Autodesk Inventor part; units mm, degrees
ref_plane "YZ Plane" through (0, 0, 0) normal (1, 0, 0) x (0, 1, 0)
ref_plane "XZ Plane" through (0, 0, 0) normal (0, 1, 0) x (-1, 0, 0)
ref_plane "XY Plane" through (0, 0, 0) normal (0, 0, 1) x (1, 0, 0)
sketch "Sketch1" plane through (0, 0, 0) normal (0, 0, 1) x (1, 0, 0)
  line L0 (0, 0) -> (0, 39.4806) construction
  line L1 (0, 0) -> (-3, 0) construction
  line L2 (-3, 0) -> (-3, 27)
  line L3 (-3, 27) -> (-5, 27)
  line L4 (-5, 27) -> (-5, 28.75)
  line L5 (0, 0) -> (0, 29)
  line L6 (-3, 0) -> (-2.65, 0)
  line L7 (-2.65, -1.5) -> (0, -1.5)
  line L8 (0, -1.5) -> (0, 0)
  line L9 (-2.65, 0) -> (-2.65, -1.5)
  line L10 (-5, 28.75) -> (0, 28.75)
  dimension "d0" = 3
  dimension "d1" = 5
  dimension "d5" = 27
  dimension "d12" = 2.65
  dimension "d13" = 1.5
  dimension "d24" = 1.75
revolve "Revolution1" add sketch "Sketch1" angle 360 about axis through (0, 0, 0) along (0, 1, 0)
sketch "Sketch3" plane through (0, -1.5, 0) normal (0, -1, 0) x (1, 0, 0)
  point P0 (0, 0)
  point P1 (0, 0)
hole "Hole1" at (0, -1.5, 0) direction (0, 1, 0) diameter 3.242 depth 11.8 tip angle 118
sketch "Sketch4" plane through (0, 27, 0) normal (0, -1, 0) x (1, 0, 0)
  arc A0 (4, 3) -> (-4, 3) centre (0, 0) ccw
  line L0 (-4, 3) -> (4, 3)
  circle A1 centre (0, 0) radius 3
  circle A2 centre (0, 0) radius 5
extrude "Extrusion2" cut sketch "Sketch4" against normal through all contours L0 A0
properties part number "shim_peg_V3"
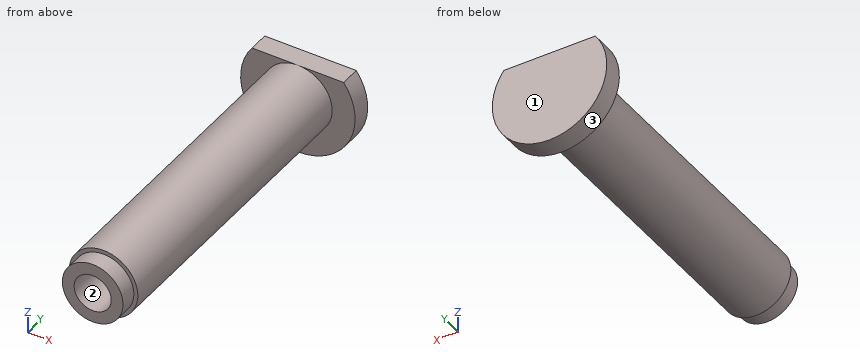
Part model, mm, in its own coordinate system. Face numbers are marked on the shaded views. Coordinates: 2 decimals unless noted, no trailing zeros. Write each loop counter-clockwise with the first axis right and the second up, starting at its lowest first coordinate (ties: lowest second). Pieces come first, ordered by that corner, then holes. Notation, with made-up numbers: M 18,-18 L 31,-18 A25 cw 31,17 Z; hole C -31,20.5 d1. An arc over 180 degrees is marked long. Return JSON: item names as keys, results as strings.
1. Saw through at C-C, the plane y = 12. Write the cut outline in (x, z).
Determined:
{"outline": "C 0,0 d6"}
2. Flat gauge pins, fed straight in: pin 1 Ø1.5 at (x, y) = (-1.5, 10) entering from +Z; pin 2 Ø5 at (x, y) = (3, 16.5) entering from -Z; pin 3 Ø2 at (x, z) = (3, -3.5) entering from -Y; pin 4 Ø2.5 at (x, z) = (1.5, 0) entering from -Y. Where does each tip first touch, or does it go through?
Determined:
{"pin 1": "z = 2.9", "pin 2": "z = -2.96", "pin 3": "y = 27", "pin 4": "y = -1.5"}
3. Saw through at A-A, the plane y = 8.5. Write the cut outline in (x, z), then the cut area to 3 significant figures.
Determined:
{"outline": "C 0,0 d6; hole C 0,0 d3.24", "area": "20.0 mm²"}
4. Pull direction Z, two halves, no side cores. Call the marked faces 1, 2 and 3: pulls with the +Z half, pulls with the -Z half, needs draft (parallel to the pull), parting line crosses it, or undercut.
Determined:
{"face 1": "needs draft", "face 2": "undercut", "face 3": "parting line crosses it"}
5. Saw through at B-B, the plane z = -4. Write the cut outline in (x, y), then the cut area to 3 significant figures.
Determined:
{"outline": "M -3,27 L 3,27 L 3,28.75 L -3,28.75 Z", "area": "10.5 mm²"}
6. Saw through at D-D, the plane x = -3.5. Write the cut outline in (y, z), then the cut area to 3 significant figures.
Determined:
{"outline": "M 27,-3.57 L 28.75,-3.57 L 28.75,3 L 27,3 Z", "area": "11.5 mm²"}
7. Probe L1, parallel to Z at x = 0, y = 5; L2, parallel to Y at x = 1.75, z = -4.5. List the from-to ranges inside material, lowest first.
Determined:
{"L1": "-3 to -1.62, 1.62 to 3", "L2": "27 to 28.75"}
